```python
from build123d import *

# Parameters (mm, degrees)
HEAD_DEPTH         = 8
HOLE_SKETCH_R      = 4
THROUGH_HOLE_DEPTH = 9


with BuildPart() as part:
    # Head Sketch → Head (new body)
    with BuildSketch(Plane.XY):
        Polygon((0, 7.505553499), (6.5, 3.75277675), (6.5, -3.75277675), (0, -7.505553499), (-6.5, -3.75277675), (-6.5, 3.75277675), align=None)
    extrude(amount=HEAD_DEPTH)

    # Flange Sketch → Flange (revolve)
    with BuildSketch(Plane(origin=(0, 0, 0), x_dir=(-1, 0, 0), z_dir=(0, 1, 0))):
        with BuildLine():
            Line((-8.95, 0), (0, 0))
            Line((0, 0), (0, 2.5))
            ThreePointArc((0, 2.5), (-4.620060107, 2.115525306), (-9.11301873, 0.972678425))
            ThreePointArc((-9.11301873, 0.972678425), (-9.443122304, 0.417353804), (-8.95, 0))
        make_face()
    revolve(axis=Axis((0, 0, 1.843425858), (0, 0, 1)))

    # Sketch5 → Head Trim (revolve, cut)
    with BuildSketch(Plane(origin=(0, 0, 0), x_dir=(0, 0, -1), z_dir=(1, 0, 0))):
        with BuildLine():
            Line((-8, -6.505553499), (-8, -7.505553499))
            Line((-8, -7.505553499), (-7, -7.505553499))
            ThreePointArc((-7, -7.505553499), (-7.707106781, -7.212660281), (-8, -6.505553499))
        make_face()
    revolve(axis=Axis((0, 0, 15.085599173), (0, 0, -1)), mode=Mode.SUBTRACT)

    # Hole Sketch → Through Hole (cut, through all)
    with BuildSketch(Plane.XY.offset(8)):
        Circle(HOLE_SKETCH_R)
    extrude(amount=-THROUGH_HOLE_DEPTH, mode=Mode.SUBTRACT)


solid = part.part
```
Work out the finished part from the listing and answer in its coordinate system (mm). A direction names the side the tool comes from. Give positions to 0.01 mm unless a question says otherwise; leave off trailing zeros. Write each loop counter-clockwise with the first axis right and the second up, starting at its lowest first coordinate (ties: lowest second). Pieces come first, ordered by that corner, then holes.
(1) The part is cut by section B-B on z = 3.75. Write down the section's boundary in (x, y).
Final values:
outline: (-6.5, -3.75) - (0, -7.51) - (6.5, -3.75) - (6.5, 3.75) - (0, 7.51) - (-6.5, 3.75) - close; hole circle Ø8 at (0, 0)
(2) Which of the six approach directions +Z, -Z, +X, -X, +Y, -Y give full straight-line access (tool end or side, diameter ignored) to faces 4 (the flat face through (3.2, 5.66, 4.69)), 5 (the flat face through (3.3, -5.6, 4.7)), 6 (the flat face through (-3.3, 5.6, 4.7))?
Final values:
face 4: +Z, +X, +Y
face 5: +Z, +X, -Y
face 6: +Z, -X, +Y
(3) The part is cut by section C-C on z = 1.25. Write down the section's boundary in (x, y).
Final values:
outline: circle Ø16.53 at (0, 0); hole circle Ø8 at (0, 0)
(4) Straight lines are drawn through the part: line 1 (Y direction, x = 2.5, z = 7); line 2 (Y direction, x = 1.25, z = 0.75); line 3 (X direction, y = 5.5, z = 3.5). For each, find the intervals that lie inside material, in ascending order.
Final values:
line 1: y = -6.06 to -3.12, 3.12 to 6.06
line 2: y = -9.3 to -3.8, 3.8 to 9.3
line 3: x = -3.47 to 3.47
(5) The mould has two halves that part along Y. Classify faces 1 (the flat face through (-3.2, -5.66, 4.69)), 2 (the flat face through (-6.5, 0, 5)), 3 (the cylindrical face through (-0.867, -3.905, 4.056)): pulls with the +Y half, pulls with the -Y half, needs draft (parallel to the pull), parting line crosses it, or undercut.
Final values:
face 1: pulls with the -Y half
face 2: needs draft
face 3: undercut
(6) Flat-ended cylindrical pins translate along their axes: pin 1 Ø2 at (y, z) = (-1, 1) entering from +X; pin 2 Ø1.5 at (x, z) = (3, 7) entering from +Y; pin 3 Ø3.5 at (y, z) = (-0.5, 6) entering from +X. Find the tip coordinate at first contact, or state that the pin passes through.
Final values:
pin 1: stops at x = 9.45
pin 2: stops at y = 6.21
pin 3: stops at x = 6.5
(7) The part is cut by section A-A on y = 0. Write down the section's boundary in (x, z), plus the area to 3 significant figures.
Final values:
outline: (-9.11, 0.97) arc R0.5 ccw to (-8.95, 0) - (-4, 0) - (-4, 8) - (-6.5, 8) - (-6.5, 1.73) arc R27.95 ccw to start; (4, 0) - (8.95, 0) arc R0.5 ccw to (9.11, 0.97) arc R27.95 ccw to (6.5, 1.73) - (6.5, 8) - (4, 8) - close
area: 47.7 mm2
